Part model, mm, in its own coordinate system. A direction names the side the tool comes from. Round coordinates to 2 decimals unless told otherwise and drop trailing zeros. Write each loop counter-clockwise with the first axis right and the second up, starting at its lowest first coordinate (ties: lowest second). Pieces come first, ordered by that corner, then holes.
1) Flat gauge pins, fed straight in: pin 1 (3 mm diameter, centred on x = 1.5, y = 0, fed in from -Z); pin 2 (12 mm diameter, centred on x = -15.5, z = 28, fed in from +Y); pin 3 (0.6 mm diameter, centred on y = -3, z = 3, fed in from +X). Where does each tip first touch, or does it go through?
2) Which spindle directions (+Z, -Z, +X, -X, +Y, -Y) get a long thin tool onto all of the face, cutting with end or side? Do faces 1 (the flat face through (-9, -4, 0)), 2 (the flat face through (-2, -2, 10.25)), 3 (the flat face through (-2, -2, 20.5)). Say none if no direction does.
3) Saw through at C-C on z = 8. Write the cut outline in (x, y).
4) Drill centre lines: L1, parallel to Z at x = -10.5, y = -3.6; L2, parallel to Y at x = 0, z = 35.25; L3, parallel to Z at x = 0.25, y = 4.25. Where is each one in solid material? Low to high.
5) Pull direction Y, two halves, no side cores. Call faces 4 (the cylindrical face through (-0.54, 2.44, 15.3)), 5 (the flat face through (-3, -1, 41)), 6 (the flat face through (-9, -4.6, 20)): +Y half, -Y half, draft (parallel to the pull), parting line (faces both ways), or undercut.
6) Saw through at A-A on z = 33. Write the cut outline in (x, y), and give its area (3 significant figures).
7) Saw through at D-D on y = 3.5. Write the cut outline in (x, z).
8) Saw through at B-B on x = -10.5. Write the cut outline in (y, z).
Autodesk Inventor part; units mm, degrees
ref_plane "3_to_1_XY" through (0, 0, 20.5) normal (0, 0, 1) x (1, 0, 0)
ref_plane "3_to_1_YZ" through (0, 0, 20.5) normal (1, 0, 0) x (0, 1, 0)
ref_plane "3_to_1_ZX" through (0, 0, 20.5) normal (0, 1, 0) x (0, 0, 1)
sketch "Sketch_1" plane through (0, 0, 0) normal (0, 0, 1) x (1, 0, 0)
  line L0 (-18, -4.6) -> (0, -4.6)
  arc A0 (0, -4.6) -> (-3.7947, -2.6) centre (0, 0) ccw
  line L1 (-3.7947, -2.6) -> (-18, -2.6)
  line L2 (-18, -2.6) -> (-18, -4.6)
  circle A1 centre (0, 0) radius 2.5
extrude "Extrusion1" add sketch "Sketch_1" along normal blind 41
sketch "Sketch_2" plane through (0, -4.6, 0) normal (0, 1, 0) x (1, 0, 0)
  line L0 (-20, 2) -> (-20, -43)
  line L1 (-20, -43) -> (-9.2, -43)
  line L2 (-9.2, -43) -> (-9.2, -41)
  line L3 (-9.2, -41) -> (-14, -41)
  arc A0 (-18, -37) -> (-14, -41) centre (-14, -37) ccw
  line L4 (-18, -37) -> (-18, -4)
  arc A1 (-14, 0) -> (-18, -4) centre (-14, -4) ccw
  line L5 (-14, 0) -> (-9.2, 0)
  line L6 (-9.2, 0) -> (-9.2, 2)
  line L7 (-9.2, 2) -> (-20, 2)
extrude "Extrusion2" cut sketch "Sketch_2" along normal blind 2
sketch "Sketch_3" plane through (0, -4.6, 0) normal (0, 1, 0) x (1, 0, 0)
  circle A0 centre (-10.5, -33) radius 2.75
extrude "Extrusion3" cut sketch "Sketch_3" along normal blind 2
sketch "Sketch_4" plane through (0, -4.6, 0) normal (0, 1, 0) x (1, 0, 0)
  circle A0 centre (-10.5, -8) radius 2.75
extrude "Extrusion4" cut sketch "Sketch_4" along normal blind 2
sketch "Sketch_7" plane through (0, 0, 0) normal (0, 0, 1) x (1, 0, 0)
  line L0 (-4.6, -4.6) -> (0, -4.6)
  arc A0 (0, -4.6) -> (-4.6, 0) centre (0, 0) ccw
  line L1 (-4.6, 0) -> (-4.6, -4.6)
extrude "Extrusion5" cut sketch "Sketch_7" along normal blind 10.25
sketch "Sketch_5" plane through (0, 0, 30.75) normal (0, 0, 1) x (1, 0, 0)
  line L0 (-4.6, -4.6) -> (0, -4.6)
  arc A0 (0, -4.6) -> (-4.6, 0) centre (0, 0) ccw
  line L1 (-4.6, 0) -> (-4.6, -4.6)
extrude "Extrusion6" cut sketch "Sketch_5" against normal blind 10.25
ref_plane "3_to_1_XY" through (0, 0, 20.5) normal (0, 0, 1) x (1, 0, 0)
ref_plane "3_to_1_YZ" through (0, 0, 20.5) normal (1, 0, 0) x (0, 1, 0)
ref_plane "3_to_1_ZX" through (0, 0, 20.5) normal (0, 1, 0) x (0, 0, 1)
properties part number "SHPSNA5_3"
Completed:
1. pin 1: stops at z = 10.25
1. pin 2: stops at y = -2.6
1. pin 3: stops at x = -4.6
2. face 1: -Z, +X, -X, +Y, -Y
2. face 2: -Z, +X, +Y, -Y
2. face 3: +X, +Y, -Y
3. outline: (-18, -4.6) - (-13.25, -4.6) - (-13.25, -2.6) - (-18, -2.6) - close; (-7.75, -4.6) - (-4.6, -4.6) - (-4.6, -2.6) - (-7.75, -2.6) - close
4. L1: z = 0 to 5.25, 10.75 to 30.25, 35.75 to 41
4. L2: y = -4.6 to -2.5, 2.5 to 4.6
4. L3: z = 10.25 to 20.5, 30.75 to 41
5. face 4: undercut
5. face 5: draft
5. face 6: -Y half
6. outline: (-18, -4.6) - (-13.25, -4.6) - (-13.25, -2.6) - (-18, -2.6) - close; (-7.75, -4.6) - (0, -4.6) arc R4.6 ccw (long way) to (-3.79, -2.6) - (-7.75, -2.6) - close; hole circle Ø5 at (0, 0)
6. area: 66.5 mm2
7. outline: (-2.98, 10.25) - (2.98, 10.25) - (2.98, 20.5) - (-2.98, 20.5) - close; (-2.98, 30.75) - (2.98, 30.75) - (2.98, 41) - (-2.98, 41) - close
8. outline: (-4.6, 0) - (-2.6, 0) - (-2.6, 5.25) - (-4.6, 5.25) - close; (-4.6, 10.75) - (-2.6, 10.75) - (-2.6, 30.25) - (-4.6, 30.25) - close; (-4.6, 35.75) - (-2.6, 35.75) - (-2.6, 41) - (-4.6, 41) - close
